from build123d import *

# Parameters (mm, degrees)
SKETCH1_W                  = 1.5
SKETCH1_H                  = 0.75
BOSS_EXTRUDE1_DEPTH        = 1.875
BOSS_EXTRUDE1_DEPTH_BACK   = 0.625
FILLET1_R                  = 0.5
F_0_4_0_4_DIAMETER_HOLE1_D = 0.4


with BuildPart() as part:
    # Sketch1 → Boss-Extrude1 (new body, two sides)
    with BuildSketch(Plane.XY) as boss_extrude1_sk:
        Polygon((0.285769435, 0.25), (-1.464230565, 0.25), (-1.464230565, -5), (-1.464230565, -5.75), (0.285769435, -5.75), align=None)
        Polygon((-1.464230565, 2), (-1.464230565, 0.25), (0.285769435, 0.25), (1.535769435, 0.25), (1.535769435, 2), align=None)
        with Locations((-2.214230565, -5.375)):
            Rectangle(SKETCH1_W, SKETCH1_H)
    extrude(amount=BOSS_EXTRUDE1_DEPTH)
    extrude(boss_extrude1_sk.sketch, amount=-BOSS_EXTRUDE1_DEPTH_BACK)

    # Fillet1
    fillet1_edges = [part.edges().sort_by_distance(p)[0] for p in [
        (0.285769435, 0.25, 0.625),
        (-2.964230565, -5, 0.625),
        (-1.464230565, -5, 0.625),
        (0.285769435, -5.75, 0.625),
        (-1.464230565, 2, 0.625),
    ]]
    fillet(fillet1_edges, radius=FILLET1_R)

    # Ø0.4 (0.4) Diameter Hole1 (through all)
    with Locations(Plane(origin=(0, -5, 0), x_dir=(1, 0, 0), z_dir=(0, 1, 0))):
        with Locations((-2.214230565, 0), (-2.214230565, -1.25)):
            Hole(F_0_4_0_4_DIAMETER_HOLE1_D / 2)


solid = part.part
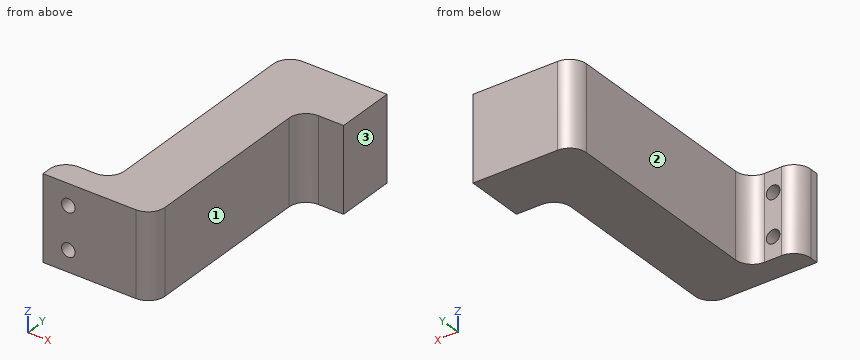
Source: CAD feature listing. Evaluate the final solid. Frame: model axes, mm. Face numbers are marked on the shaded views. A direction names the side the tool comes from. Round coordinates to 2 decimals unless told otherwise and drop trailing zeros. Loops run counter-clockwise (first coordinate to the right, second up) from the corner with the lowest first, then second, coordinate; pieces in that order, holes last. Notation, with made-up numbers: (57, 27) - (90, 27) arc R10 cw to (90, 39) - close; hole circle Ø2 at (12.5, -39). An arc over 180 degrees is marked (long way). Write item = value, one per line. Start each with the question number.
(1) Section query A-A, the plane z = 0. Output: boundary loops of the cut face in (x, y), plus the area to 3 significant figures.
(2) Section query C-C, the plane y = -3.75. Output: boundary loops of the cut face in (x, z) (3 decimals).
(3) Pin query (flat end, axial travel): pin 1 (1 mm diameter, centred on y = -0.5, z = 1.5, fed in from +X). Return the tip coordinate at first contact, or that it passes through.
(4) Set-up query: the marked faces 1, 2 and 3. Return all of +Z, -Z, +X, -X, +Y, -Y with unobstructed straight access to the full face (end or side cutting, diameter ignored); none if empty.
(5) Ray query, line 1 along Y through (x, z) = (1.15, 0.2); line 2 along Y through (x, z) = (-2.4, 0.6); line 3 along X through (y, z) = (-3, 1.4). Return the intervals inside material, ascending. Write a range as from..to.
(6) Section query D-D, the plane x = 1.15. Output: boundary loops of the cut face in (y, z) (3 decimals), plus the area to 4 significant figures.
(7) Section query B-B, the plane x = -2.1. Output: boundary loops of the cut face in (y, z) (3 decimals), plus the area to 3 significant figures.
Conclusion:
q1.outline = (-2.96, -5.75) - (-2.41, -5.75) - (-2.41, -5) - (-2.46, -5) arc R0.5 ccw to (-2.96, -5.5) - close; (-2.01, -5.75) - (-0.21, -5.75) arc R0.5 ccw to (0.29, -5.25) - (0.29, -0.25) arc R0.5 cw to (0.79, 0.25) - (1.54, 0.25) - (1.54, 2) - (-0.96, 2) arc R0.5 ccw to (-1.46, 1.5) - (-1.46, -4.5) arc R0.5 cw to (-1.96, -5) - (-2.01, -5) - close
q1.area = 16.5 mm2
q2.outline = (-1.464, -0.625) - (0.286, -0.625) - (0.286, 1.875) - (-1.464, 1.875) - close
q3.pin_1 = 0.35
q4.face_1 = +Z, -Z, +X, -Y
q4.face_2 = +Z, -Z, -X, +Y
q4.face_3 = +Z, -Z, +X, +Y, -Y
q5.line_1 = 0.25..2
q5.line_2 = -5.75..-5
q5.line_3 = -1.46..0.29
q6.outline = (0.25, -0.625) - (2, -0.625) - (2, 1.875) - (0.25, 1.875) - close
q6.area = 4.375 mm2
q7.outline = (-5.75, -0.625) - (-5, -0.625) - (-5, -0.164) - (-5.75, -0.164) - close; (-5.75, 0.164) - (-5, 0.164) - (-5, 1.086) - (-5.75, 1.086) - close; (-5.75, 1.414) - (-5, 1.414) - (-5, 1.875) - (-5.75, 1.875) - close
q7.area = 1.38 mm2
